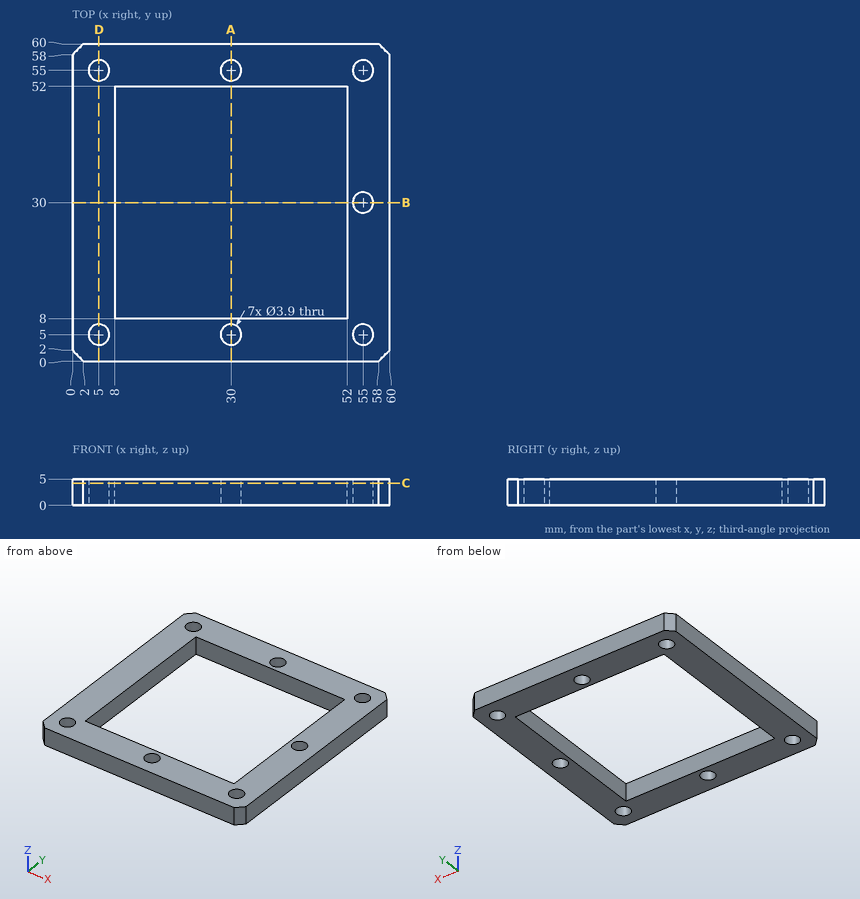
Study the drawing (mm; zero at the part's minimum x, y, z) and answer. Give positions to 0.01 mm unless a question says otherwise; leave off trailing zeros. Order: outer loops, then holes, each group sorted by start corner. A loop starts at its lowest first (then second) coordinate and runs counter-clockwise, first axis right, second up. Notation, with made-up numbers: (62.5, 74) -> (72.5, 74) arc R13 ccw to (72.5, 84) -> close; hole circle Ø6 at (64.25, 44.5). An arc over 180 degrees is marked (long way). Write item = value, one per line.
1. A cutting plane is placed at B-B, the plane y = 30. Write down the section's boundary in (x, z).
Numbers:
outline = (0, 0) -> (8, 0) -> (8, 5) -> (0, 5) -> close; (52, 0) -> (53.05, 0) -> (53.05, 5) -> (52, 5) -> close; (56.95, 0) -> (60, 0) -> (60, 5) -> (56.95, 5) -> close
2. A cutting plane is placed at D-D, the plane x = 5. Write down the section's boundary in (y, z), and give its area (3 significant figures).
Numbers:
outline = (0, 0) -> (3.05, 0) -> (3.05, 5) -> (0, 5) -> close; (6.95, 0) -> (53.05, 0) -> (53.05, 5) -> (6.95, 5) -> close; (56.95, 0) -> (60, 0) -> (60, 5) -> (56.95, 5) -> close
area = 261 mm²
3. A cutting plane is placed at A-A, the plane x = 30. Write down the section's boundary in (y, z), and give its area (3 significant figures).
Numbers:
outline = (0, 0) -> (3.05, 0) -> (3.05, 5) -> (0, 5) -> close; (6.95, 0) -> (8, 0) -> (8, 5) -> (6.95, 5) -> close; (52, 0) -> (53.05, 0) -> (53.05, 5) -> (52, 5) -> close; (56.95, 0) -> (60, 0) -> (60, 5) -> (56.95, 5) -> close
area = 41.0 mm²
4. Straight lines are drawn through the part: line 1 along Y through (x, z) = (55, 2.2); line 2 along Y through (x, z) = (30, 1.4); line 3 along Y through (x, z) = (19, 4.5). For each, find the intervals that lie inside material, in ascending order.
Numbers:
line_1 = 0 to 3.05, 6.95 to 28.05, 31.95 to 53.05, 56.95 to 60
line_2 = 0 to 3.05, 6.95 to 8, 52 to 53.05, 56.95 to 60
line_3 = 0 to 8, 52 to 60
5. A cutting plane is placed at C-C, the plane z = 4.2. Count the separate pieces of the cut face and the enclosed holes in it, and give its area (3 significant figures).
Numbers:
separate_pieces = 1
enclosed_holes = 8
area = 1,570 mm²
